Part model, mm, in its own coordinate system. A direction names the side the tool comes from. Give positions to 0.01 mm unless a question says otherwise; leave off trailing zeros. Order: outer loops, then holes, each group sorted by start corner. A loop starts at its lowest first (then second) coordinate and runs counter-clockwise, first axis right, second up. Notation, with made-up numbers: (70, 36.5) - (116, 36.5) arc R25 cw to (116, 73.5) - close; hole circle Ø11 at (72, -3). An arc over 180 degrees is marked (long way). Use a Markdown table: item, result. Add a question column.
from build123d import *

# Parameters (mm, degrees)
BASE_FLANGE1_START              = -0.9
BASE_FLANGE1_DEPTH              = 0.9
EDGE_FLANGE1_STRIP_W            = 5.6
EDGE_FLANGE1_STRIP_H            = 0.9
EDGE_FLANGE1_STRIP_CUT_DEPTH    = 80.2
EDGE_FLANGE1_RELIEF_W           = 6.05
EDGE_FLANGE1_RELIEF_H           = 0.45
EDGE_FLANGE1_RELIEF_CUT_DEPTH   = 0.9
EDGE_FLANGE1_STRIP_2_W          = 5.6
EDGE_FLANGE1_STRIP_2_H          = 0.9
EDGE_FLANGE1_STRIP_CUT_2_DEPTH  = 80.2
EDGE_FLANGE1_RELIEF_2_W         = 6.05
EDGE_FLANGE1_RELIEF_2_H         = 0.45
EDGE_FLANGE1_RELIEF_CUT_2_DEPTH = 0.9
EDGE_FLANGE1_STRIP_3_W          = 5.6
EDGE_FLANGE1_STRIP_3_H          = 0.9
EDGE_FLANGE1_STRIP_CUT_3_DEPTH  = 80.2
EDGE_FLANGE1_RELIEF_3_W         = 6.05
EDGE_FLANGE1_RELIEF_3_H         = 0.45
EDGE_FLANGE1_RELIEF_CUT_3_DEPTH = 0.9
EDGE_FLANGE1_STRIP_4_W          = 5.6
EDGE_FLANGE1_STRIP_4_H          = 0.9
EDGE_FLANGE1_STRIP_CUT_4_DEPTH  = 80.2
EDGE_FLANGE1_RELIEF_4_W         = 6.05
EDGE_FLANGE1_RELIEF_4_H         = 0.45
EDGE_FLANGE1_RELIEF_CUT_4_DEPTH = 0.9
EDGE_FLANGE1_DEPTH              = 80.2
EDGE_FLANGE1_BEND_DEPTH         = 80.2
EDGE_FLANGE1_BEND_2_DEPTH       = 80.2
EDGE_FLANGE1_BEND_3_DEPTH       = 80.2
SKETCH18_R                      = 5
CUT_EXTRUDE1_DEPTH              = 10
M2X0_4_TAPPED_HOLE1_D           = 1.6
M2X0_4_TAPPED_HOLE1_DEPTH       = 5.2
M2X0_4_TAPPED_HOLE1_TIP         = 0.480688495
M2X0_4_TAPPED_HOLE2_D           = 1.6
M2X0_4_TAPPED_HOLE2_DEPTH       = 5.2
M2X0_4_TAPPED_HOLE2_TIP         = 0.480688495
M2X0_4_TAPPED_HOLE3_D           = 1.6
M2X0_4_TAPPED_HOLE3_DEPTH       = 5.2
M2X0_4_TAPPED_HOLE3_TIP         = 0.480688495
M2X0_4_TAPPED_HOLE4_D           = 1.6
M2X0_4_TAPPED_HOLE4_DEPTH       = 5.2
M2X0_4_TAPPED_HOLE4_TIP         = 0.480688495
M4_CLEARANCE_HOLE1_D            = 4.5


# Read off the part's stored shape, not the designer's step: Base-Flange1
# Sheet-metal steps are written as plain solids
with BuildPart() as part:
    # Base-Flange1 outline → Base-Flange1 (new body)
    with BuildSketch(Plane(origin=(0, 0, 0), x_dir=(1, 0, 0), z_dir=(0, 1, 0)).offset(BASE_FLANGE1_START)):
        Polygon((98.2, 89.2), (89.2, 98.2), (9, 98.2), (0, 89.2), (0, 9), (9, 0), (89.2, 0), (98.2, 9), align=None)
    extrude(amount=BASE_FLANGE1_DEPTH)

    # Edge-Flange1 strip (across the edge) → Edge-Flange1 strip cut (cut)
    with BuildSketch(Plane(origin=(98.2, -0.9, -89.2), x_dir=(-1, 0, 0), z_dir=(0, 0, 1))):
        with Locations((-0.9, -0.45)):
            Rectangle(EDGE_FLANGE1_STRIP_W, EDGE_FLANGE1_STRIP_H)
    extrude(amount=EDGE_FLANGE1_STRIP_CUT_DEPTH, mode=Mode.SUBTRACT)

    # Edge-Flange1 relief (on the sheet) → Edge-Flange1 relief cut (cut)
    with BuildSketch(Plane(origin=(96.3, -0.9, -89.2), x_dir=(-1, 0, 0), z_dir=(0, -1, 0))):
        with Locations((-2.575, 0.225)):
            Rectangle(EDGE_FLANGE1_RELIEF_W, EDGE_FLANGE1_RELIEF_H)
        with Locations((-2.575, -80.425)):
            Rectangle(EDGE_FLANGE1_RELIEF_W, EDGE_FLANGE1_RELIEF_H)
    extrude(amount=-EDGE_FLANGE1_RELIEF_CUT_DEPTH, mode=Mode.SUBTRACT)

    # Edge-Flange1 strip 2 (across the edge) → Edge-Flange1 strip cut 2 (cut)
    with BuildSketch(Plane(origin=(89.2, -0.9, 0), x_dir=(0, 0, -1), z_dir=(-1, 0, 0))):
        with Locations((-0.9, -0.45)):
            Rectangle(EDGE_FLANGE1_STRIP_2_W, EDGE_FLANGE1_STRIP_2_H)
    extrude(amount=EDGE_FLANGE1_STRIP_CUT_2_DEPTH, mode=Mode.SUBTRACT)

    # Edge-Flange1 relief 2 (on the sheet) → Edge-Flange1 relief cut 2 (cut)
    with BuildSketch(Plane(origin=(89.2, -0.9, -1.9), x_dir=(0, 0, -1), z_dir=(0, -1, 0))):
        with Locations((-2.575, 0.225)):
            Rectangle(EDGE_FLANGE1_RELIEF_2_W, EDGE_FLANGE1_RELIEF_2_H)
        with Locations((-2.575, -80.425)):
            Rectangle(EDGE_FLANGE1_RELIEF_2_W, EDGE_FLANGE1_RELIEF_2_H)
    extrude(amount=-EDGE_FLANGE1_RELIEF_CUT_2_DEPTH, mode=Mode.SUBTRACT)

    # Edge-Flange1 strip 3 (across the edge) → Edge-Flange1 strip cut 3 (cut)
    with BuildSketch(Plane(origin=(0, -0.9, -9), x_dir=(1, 0, 0), z_dir=(0, 0, -1))):
        with Locations((-0.9, -0.45)):
            Rectangle(EDGE_FLANGE1_STRIP_3_W, EDGE_FLANGE1_STRIP_3_H)
    extrude(amount=EDGE_FLANGE1_STRIP_CUT_3_DEPTH, mode=Mode.SUBTRACT)

    # Edge-Flange1 relief 3 (on the sheet) → Edge-Flange1 relief cut 3 (cut)
    with BuildSketch(Plane(origin=(1.9, -0.9, -9), x_dir=(1, 0, 0), z_dir=(0, -1, 0))):
        with Locations((-2.575, 0.225)):
            Rectangle(EDGE_FLANGE1_RELIEF_3_W, EDGE_FLANGE1_RELIEF_3_H)
        with Locations((-2.575, -80.425)):
            Rectangle(EDGE_FLANGE1_RELIEF_3_W, EDGE_FLANGE1_RELIEF_3_H)
    extrude(amount=-EDGE_FLANGE1_RELIEF_CUT_3_DEPTH, mode=Mode.SUBTRACT)

    # Edge-Flange1 strip 4 (across the edge) → Edge-Flange1 strip cut 4 (cut)
    with BuildSketch(Plane(origin=(9, -0.9, -98.2), x_dir=(0, 0, 1), z_dir=(1, 0, 0))):
        with Locations((-0.9, -0.45)):
            Rectangle(EDGE_FLANGE1_STRIP_4_W, EDGE_FLANGE1_STRIP_4_H)
    extrude(amount=EDGE_FLANGE1_STRIP_CUT_4_DEPTH, mode=Mode.SUBTRACT)

    # Edge-Flange1 relief 4 (on the sheet) → Edge-Flange1 relief cut 4 (cut)
    with BuildSketch(Plane(origin=(9, -0.9, -96.3), x_dir=(0, 0, 1), z_dir=(0, -1, 0))):
        with Locations((-2.575, 0.225)):
            Rectangle(EDGE_FLANGE1_RELIEF_4_W, EDGE_FLANGE1_RELIEF_4_H)
        with Locations((-2.575, -80.425)):
            Rectangle(EDGE_FLANGE1_RELIEF_4_W, EDGE_FLANGE1_RELIEF_4_H)
    extrude(amount=-EDGE_FLANGE1_RELIEF_CUT_4_DEPTH, mode=Mode.SUBTRACT)

    # Edge-Flange1 section (across the edge) → Edge-Flange1 (add)
    with BuildSketch(Plane(origin=(98.2, -0.9, -89.2), x_dir=(-1, 0, 0), z_dir=(0, 0, 1))):
        with BuildLine():
            Line((0, 1), (0, 9.1))
            Line((0, 9.1), (0.9, 9.1))
            Line((0.9, 9.1), (0.9, 1))
            ThreePointArc((0.9, 1), (1.192893219, 0.292893219), (1.9, 0))
            Line((1.9, 0), (1.9, -0.9))
            ThreePointArc((1.9, -0.9), (0.556497116, -0.343502884), (0, 1))
        make_face()
    extrude(amount=EDGE_FLANGE1_DEPTH)

    # Edge-Flange1 section 2 (across the edge) → Edge-Flange1 bend (add)
    with BuildSketch(Plane(origin=(89.2, -0.9, 0), x_dir=(0, 0, -1), z_dir=(-1, 0, 0))):
        with BuildLine():
            Line((0, 1), (0, 9.1))
            Line((0, 9.1), (0.9, 9.1))
            Line((0.9, 9.1), (0.9, 1))
            ThreePointArc((0.9, 1), (1.192893219, 0.292893219), (1.9, 0))
            Line((1.9, 0), (1.9, -0.9))
            ThreePointArc((1.9, -0.9), (0.556497116, -0.343502884), (0, 1))
        make_face()
    extrude(amount=EDGE_FLANGE1_BEND_DEPTH)

    # Edge-Flange1 section 3 (across the edge) → Edge-Flange1 bend 2 (add)
    with BuildSketch(Plane(origin=(0, -0.9, -9), x_dir=(1, 0, 0), z_dir=(0, 0, -1))):
        with BuildLine():
            Line((0, 1), (0, 9.1))
            Line((0, 9.1), (0.9, 9.1))
            Line((0.9, 9.1), (0.9, 1))
            ThreePointArc((0.9, 1), (1.192893219, 0.292893219), (1.9, 0))
            Line((1.9, 0), (1.9, -0.9))
            ThreePointArc((1.9, -0.9), (0.556497116, -0.343502884), (0, 1))
        make_face()
    extrude(amount=EDGE_FLANGE1_BEND_2_DEPTH)

    # Edge-Flange1 section 4 (across the edge) → Edge-Flange1 bend 3 (add)
    with BuildSketch(Plane(origin=(9, -0.9, -98.2), x_dir=(0, 0, 1), z_dir=(1, 0, 0))):
        with BuildLine():
            Line((0, 1), (0, 9.1))
            Line((0, 9.1), (0.9, 9.1))
            Line((0.9, 9.1), (0.9, 1))
            ThreePointArc((0.9, 1), (1.192893219, 0.292893219), (1.9, 0))
            Line((1.9, 0), (1.9, -0.9))
            ThreePointArc((1.9, -0.9), (0.556497116, -0.343502884), (0, 1))
        make_face()
    extrude(amount=EDGE_FLANGE1_BEND_3_DEPTH)

    # Sketch18 → Cut-Extrude1 (cut)
    with BuildSketch(Plane(origin=(0, 0, 0), x_dir=(1, 0, 0), z_dir=(0, 1, 0))):
        with Locations(Location((49.1, 49.1, 0), (0, 0, 270))):
            Circle(SKETCH18_R)
        with BuildLine():
            Line((70.557864376, 8.5), (27.642135624, 8.5))
            ThreePointArc((27.642135624, 8.5), (23.022737961, 11.586582838), (24.106601718, 17.035533906))
            Line((24.106601718, 17.035533906), (44.534608033, 37.463540221))
            ThreePointArc((44.534608033, 37.463540221), (49.1, 36.6), (53.665391967, 37.463540221))
            Line((53.665391967, 37.463540221), (74.093398282, 17.035533906))
            ThreePointArc((74.093398282, 17.035533906), (75.177262039, 11.586582838), (70.557864376, 8.5))
        make_face()
        with BuildLine():
            Line((8.5, 27.642135624), (8.5, 70.557864376))
            ThreePointArc((8.5, 70.557864376), (11.586582838, 75.177262039), (17.035533906, 74.093398282))
            Line((17.035533906, 74.093398282), (37.463540221, 53.665391967))
            ThreePointArc((37.463540221, 53.665391967), (36.6, 49.1), (37.463540221, 44.534608033))
            Line((37.463540221, 44.534608033), (17.035533906, 24.106601718))
            ThreePointArc((17.035533906, 24.106601718), (11.586582838, 23.022737961), (8.5, 27.642135624))
        make_face()
        with BuildLine():
            Line((27.642135624, 89.7), (70.557864376, 89.7))
            ThreePointArc((70.557864376, 89.7), (75.177262039, 86.613417162), (74.093398282, 81.164466094))
            Line((74.093398282, 81.164466094), (53.665391967, 60.736459779))
            ThreePointArc((53.665391967, 60.736459779), (49.1, 61.6), (44.534608033, 60.736459779))
            Line((44.534608033, 60.736459779), (24.106601718, 81.164466094))
            ThreePointArc((24.106601718, 81.164466094), (23.022737961, 86.613417162), (27.642135624, 89.7))
        make_face()
        with BuildLine():
            Line((89.7, 70.557864376), (89.7, 27.642135624))
            ThreePointArc((89.7, 27.642135624), (86.613417162, 23.022737961), (81.164466094, 24.106601718))
            Line((81.164466094, 24.106601718), (60.736459779, 44.534608033))
            ThreePointArc((60.736459779, 44.534608033), (61.6, 49.1), (60.736459779, 53.665391967))
            Line((60.736459779, 53.665391967), (81.164466094, 74.093398282))
            ThreePointArc((81.164466094, 74.093398282), (86.613417162, 75.177262039), (89.7, 70.557864376))
        make_face()
    extrude(amount=-CUT_EXTRUDE1_DEPTH, mode=Mode.SUBTRACT)

    # M2x0.4 Tapped Hole1
    with Locations(Plane(origin=(98.2, -86.276184469, 4.184287404), x_dir=(0, 0, 1), z_dir=(1, 0, 0))):
        with Locations((-83.284287404, -82.026184469), (-53.284287404, -82.026184469), (-23.284287404, -82.026184469)):
            Hole(M2X0_4_TAPPED_HOLE1_D / 2, depth=M2X0_4_TAPPED_HOLE1_DEPTH)
            with Locations((0, 0, -(M2X0_4_TAPPED_HOLE1_DEPTH + M2X0_4_TAPPED_HOLE1_TIP / 2))):  # 118° drill point
                Cone(0, M2X0_4_TAPPED_HOLE1_D / 2, M2X0_4_TAPPED_HOLE1_TIP, mode=Mode.SUBTRACT)

    # M2x0.4 Tapped Hole2
    with Locations(Plane(origin=(24.191898312, -86.276184469, -98.2), x_dir=(1, 0, 0), z_dir=(0, 0, -1))):
        with Locations((-5.091898312, -82.026184469), (24.908101688, -82.026184469), (54.908101688, -82.026184469)):
            Hole(M2X0_4_TAPPED_HOLE2_D / 2, depth=M2X0_4_TAPPED_HOLE2_DEPTH)
            with Locations((0, 0, -(M2X0_4_TAPPED_HOLE2_DEPTH + M2X0_4_TAPPED_HOLE2_TIP / 2))):  # 118° drill point
                Cone(0, M2X0_4_TAPPED_HOLE2_D / 2, M2X0_4_TAPPED_HOLE2_TIP, mode=Mode.SUBTRACT)

    # M2x0.4 Tapped Hole3
    with Locations(Plane(origin=(0, -86.276184469, 4.184287404), x_dir=(0, 0, -1), z_dir=(-1, 0, 0))):
        with Locations((83.284287404, -82.026184469), (53.284287404, -82.026184469), (23.284287404, -82.026184469)):
            Hole(M2X0_4_TAPPED_HOLE3_D / 2, depth=M2X0_4_TAPPED_HOLE3_DEPTH)
            with Locations((0, 0, -(M2X0_4_TAPPED_HOLE3_DEPTH + M2X0_4_TAPPED_HOLE3_TIP / 2))):  # 118° drill point
                Cone(0, M2X0_4_TAPPED_HOLE3_D / 2, M2X0_4_TAPPED_HOLE3_TIP, mode=Mode.SUBTRACT)

    # M2x0.4 Tapped Hole4
    with Locations(Plane(origin=(24.191898312, -86.276184469, 0), x_dir=(-1, 0, 0), z_dir=(0, 0, 1))):
        with Locations((-24.908101688, -82.026184469), (5.091898312, -82.026184469), (-54.908101688, -82.026184469)):
            Hole(M2X0_4_TAPPED_HOLE4_D / 2, depth=M2X0_4_TAPPED_HOLE4_DEPTH)
            with Locations((0, 0, -(M2X0_4_TAPPED_HOLE4_DEPTH + M2X0_4_TAPPED_HOLE4_TIP / 2))):  # 118° drill point
                Cone(0, M2X0_4_TAPPED_HOLE4_D / 2, M2X0_4_TAPPED_HOLE4_TIP, mode=Mode.SUBTRACT)

    # M4 Clearance Hole1 (through all)
    with Locations(Plane(origin=(24.191898312, -0.9, 4.184287404), x_dir=(0, 0, 1), z_dir=(0, -1, 0))):
        with Locations((-92.284287404, 14.091898312), (-92.284287404, -63.908101688), (-14.284287404, -63.908101688), (-14.284287404, 14.091898312)):
            Hole(M4_CLEARANCE_HOLE1_D / 2)


solid = part.part
1. Tool access for faces 1 (the face through (93.6, -0.5, -4.4)), 2 (the face through (11.511, -0.444, -75.145)), 3 (the face through (98, -4, -9)), 4 (the face through (50, -6, -0.9)): list every direction of +Z, -Z, +X, -X, +Y, -Y with a clear straight run to the whole face (end or side of a thin tool).
2. Cut at B-B (x = 58.5). Write the cut outline in (y, z), plus the area to 3 significant figures.
3. Drill centre lines: probe 1 along X at (y, z) = (-4.25, -0.7); probe 2 along Z at (x, y) = (98, -4.25); probe 3 along X at (y, z) = (-6.25, -36.5). Where is each one in solid material? Low to high. Write a range as [from, to].
4. Cut at C-C (z = -29). Write the cut outline in (x, y), plus the area to 3 significant figures.
5. Mould opens along Z. For faces 5 (the face through (9, -4, -98)), 6 (the face through (75.208, -0.444, -11.663)), 7 (the face through (4.4, -0.5, -4.6)) say: released by +Z, released by -Z, zero draft, split by the parting line, or undercut.
6. Pin check, flat tips, straight feed: P1, Ø1, axis at x = 49.1, y = -4.25, coming from the +Z side; P2, Ø4, axis at x = 53, z = -37, coming from the -Y side; P3, Ø1, axis at x = 45.5, y = -0.5, coming from the +Z side; P4, Ø0.7, axis at y = -0.5, z = -96.5, coming from the -X side. Stop position of each tip, or through.
7. Cut at A-A (y = -8.5). Write the cut outline in (x, z), plus the area to 3 significant figures.
8. Cut at D-D (x = 47). Write the cut outline in (y, z), plus the area to 3 significant figures.
Responses:
| question | item | result |
|---|---|---|
| 1 | face 1 | +Z, +X, +Y, -Y |
| 1 | face 2 | +Y, -Y |
| 1 | face 3 | +X, +Y, -Y |
| 1 | face 4 | +X, -X, -Y |
| 2 | outline | (-10, -98.2) - (-1.9, -98.2) arc R1.9 ccw to (0, -96.3) - (0, -89.7) - (-0.9, -89.7) - (-0.9, -96.3) arc R1 cw to (-1.9, -97.3) - (-10, -97.3) - close; (-10, -0.9) - (-1.9, -0.9) arc R1 cw to (-0.9, -1.9) - (-0.9, -8.5) - (0, -8.5) - (0, -1.9) arc R1.9 ccw to (-1.9, 0) - (-10, 0) - close; (-0.9, -65.57) - (0, -65.57) - (0, -32.63) - (-0.9, -32.63) - close |
| 2 | area | 60.2 mm² |
| 3 | probe 1 | x = [9, 18.3], [19.9, 48.3], [49.9, 78.3], [79.9, 89.2] |
| 3 | probe 2 | z = [-89.2, -79.9], [-78.3, -49.9], [-48.3, -19.9], [-18.3, -9] |
| 3 | probe 3 | x = [0, 0.9], [97.3, 98.2] |
| 4 | outline | (0, -10) - (0.9, -10) - (0.9, -1.9) arc R1 cw to (1.9, -0.9) - (8.5, -0.9) - (8.5, 0) - (1.9, 0) arc R1.9 ccw to (0, -1.9) - close; (21.93, -0.9) - (36.07, -0.9) - (36.07, 0) - (21.93, 0) - close; (62.13, -0.9) - (76.27, -0.9) - (76.27, 0) - (62.13, 0) - close; (89.7, -0.9) - (96.3, -0.9) arc R1 cw to (97.3, -1.9) - (97.3, -10) - (98.2, -10) - (98.2, -1.9) arc R1.9 ccw to (96.3, 0) - (89.7, 0) - close |
| 4 | area | 56.0 mm² |
| 5 | face 5 | zero draft |
| 5 | face 6 | undercut |
| 5 | face 7 | released by +Z |
| 6 | P1 | passes through |
| 6 | P2 | stops at y = -0.9 |
| 6 | P3 | stops at z = -0.23 |
| 6 | P4 | stops at x = 6.95 |
| 7 | outline | (0, -89.2) - (0.9, -89.2) - (0.9, -9) - (0, -9) - close; (9, -98.2) - (89.2, -98.2) - (89.2, -97.3) - (9, -97.3) - close; (9, -0.9) - (89.2, -0.9) - (89.2, 0) - (9, 0) - close; (97.3, -89.2) - (98.2, -89.2) - (98.2, -9) - (97.3, -9) - close |
| 7 | area | 289 mm² |
| 8 | outline | (-10, -98.2) - (-1.9, -98.2) arc R1.9 ccw to (0, -96.3) - (0, -89.7) - (-0.9, -89.7) - (-0.9, -96.3) arc R1 cw to (-1.9, -97.3) - (-10, -97.3) - close; (-10, -0.9) - (-1.9, -0.9) arc R1 cw to (-0.9, -1.9) - (-0.9, -8.5) - (0, -8.5) - (0, -1.9) arc R1.9 ccw to (-1.9, 0) - (-10, 0) - close; (-0.9, -61.42) - (0, -61.42) - (0, -53.64) - (-0.9, -53.64) - close; (-0.9, -44.56) - (0, -44.56) - (0, -36.78) - (-0.9, -36.78) - close |
| 8 | area | 44.6 mm² |
